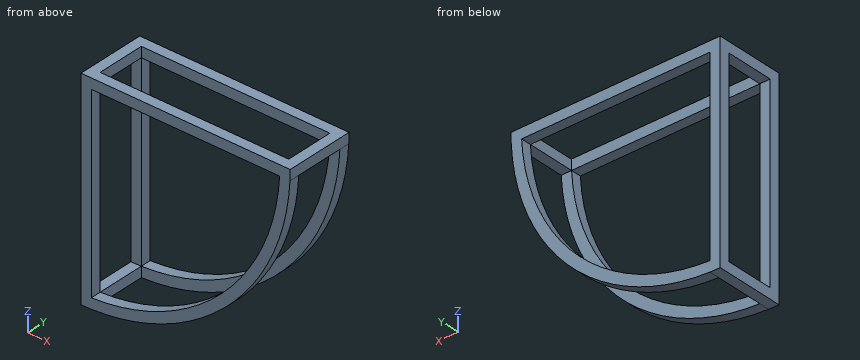
```python
from build123d import *

# Parameters (mm, degrees)
F0_W     = 6
F0_H     = 6
F1_DEPTH = 26
F2_DEPTH = 6


with BuildPart() as f1:
    # F0 (on Front) → F1 (new body)
    with BuildSketch(Plane.XZ):
        with Locations((3, -3)):
            Rectangle(F0_W, F0_H)
    extrude(amount=F1_DEPTH)



with BuildPart() as f1b:
    # F0 (on Front) → F1, piece 2 (new body)
    with BuildSketch(Plane.XZ):
        with BuildLine():
            Line((120, -6), (121.3517614211, -6))
            ThreePointArc((121.3517614211, -6), (121.4629347016, -3.0009154718), (121.5, 0))
            Line((121.5, 0), (115.5, 0))
            ThreePointArc((115.5, 0), (115.4610060581, -3.0010131717), (115.3440505618, -6))
            Line((115.3440505618, -6), (120, -6))
        make_face()
    extrude(amount=F1_DEPTH)


with BuildPart() as f1c:
    # F0 (on Front) → F1, piece 3 (new body)
    with BuildSketch(Plane.XZ):
        with BuildLine():
            Line((0, -115.5), (0, -121.5))
            ThreePointArc((0, -121.5), (3.0009154718, -121.4629347016), (6, -121.3517614211))
            Line((6, -121.3517614211), (6, -120))
            Line((6, -120), (6, -115.3440505618))
            ThreePointArc((6, -115.3440505618), (3.0010131717, -115.4610060581), (0, -115.5))
        make_face()
    extrude(amount=F1_DEPTH)


with BuildPart() as f1_1:
    add(f1.part)

    add(f1b.part)  # F2 merges F1b

    add(f1c.part)  # F2 merges F1c
    # F0 (on Front) → F2 (join)
    with BuildSketch(Plane.XZ):
        with BuildLine():
            Line((6, 0), (6, -6))
            Line((6, -6), (115.3440505618, -6))
            ThreePointArc((115.3440505618, -6), (115.4610060581, -3.0010131717), (115.5, 0))
            Line((115.5, 0), (6, 0))
        make_face()
        with BuildLine():
            Line((6, -120), (6, -121.3517614211))
            ThreePointArc((6, -121.3517614211), (85.9134739142, -85.9134739142), (121.3517614211, -6))
            Line((121.3517614211, -6), (120, -6))
            Line((120, -6), (115.3440505618, -6))
            ThreePointArc((115.3440505618, -6), (81.670833227, -81.670833227), (6, -115.3440505618))
            Line((6, -115.3440505618), (6, -120))
        make_face()
        with BuildLine():
            Line((0, -6), (0, -115.5))
            ThreePointArc((0, -115.5), (3.0010131717, -115.4610060581), (6, -115.3440505618))
            Line((6, -115.3440505618), (6, -6))
            Line((6, -6), (0, -6))
        make_face()
    extrude(amount=F2_DEPTH)


with BuildPart() as f1_2:
    # F3: moved
    add(f1_1.part.moved(Location((0, 20, 0))))

    # F4: F1 across plane


with BuildPart() as f1_3:
    add(f1_2.part)
    add(f1_2.part.mirror(Plane.XZ))


solid = f1_3.part
```
Geometry: final body of the model. Coordinates: model frame, mm. Coordinates: 2 decimals unless noted, no trailing zeros. Order: outer loops, then holes, each group sorted by start corner. A loop starts at its lowest first (then second) coordinate and runs counter-clockwise, first axis right, second up. Notation, with made-up numbers: (-36.5, -31) - (-1.5, -31) arc R6 cw to (-1.5, -21) - close; hole circle Ø6 at (5.25, -24.75). An arc over 180 degrees is marked (long way). Write each question's results on one line, items separated by ' | '.
(1) Section query B-B, the plane y = -4. Return the cut outline in (x, z).
Values found:
outline: (0, -121.5) arc R121.5 ccw to (6, -121.35) - (6, -115.34) arc R115.5 cw to (0, -115.5) - close; (0, -6) - (6, -6) - (6, 0) - (0, 0) - close; (115.34, -6) - (121.35, -6) arc R121.5 ccw to (121.5, 0) - (115.5, 0) arc R115.5 cw to start
(2) Section query C-C, the plane x = 111. Return the cut outline in (y, z), plus the area to 3 significant figures.
Values found:
outline: (-20, -49.41) - (-14, -49.41) - (-14, -31.93) - (-20, -31.93) - close; (-20, -6) - (-14, -6) - (-14, 0) - (-20, 0) - close; (14, -49.41) - (20, -49.41) - (20, -31.93) - (14, -31.93) - close; (14, -6) - (20, -6) - (20, 0) - (14, 0) - close | area: 282 mm²
(3) Section query A-A, the plane z = -40. Return the cut outline in (x, y).
Values found:
outline: (0, -20) - (6, -20) - (6, -14) - (0, -14) - close; (0, 14) - (6, 14) - (6, 20) - (0, 20) - close; (108.35, -20) - (114.73, -20) - (114.73, -14) - (108.35, -14) - close; (108.35, 14) - (114.73, 14) - (114.73, 20) - (108.35, 20) - close
(4) Line query: line 1 (Y direction, x = 38, z = -5); line 2 (X direction, y = 14.5, z = -87.5); line 3 (Z direction, x = 72, y = -15). Output: solid intervals per line, ascending. Write a range as [from, to].
Values found:
line 1: y = [-20, -14], [14, 20] | line 2: x = [0, 6], [75.39, 84.3] | line 3: z = [-97.87, -90.31], [-6, 0]
(5) First-contact query: pin 1 Ø3 at (y, z) = (18, -37) entering from +X; pin 2 Ø1.8 at (y, z) = (-6.5, -119) entering from +X; pin 3 Ø8 at (x, y) = (85, -13) entering from -Z; pin 4 Ø12 at (x, y) = (95, 3) entering from -Z. Flat tips, straight axial feed; report the tip coordinate or a pass-through.
Values found:
pin 1: stops at x = 116.2 | pin 2: stops at x = 6 | pin 3: stops at z = -90.45 | pin 4: passes through
